Geometry check sheet. Reference: the model listing, model coordinates, mm. A direction names the side the tool comes from. Give positions to 0.01 mm unless a question says otherwise; leave off trailing zeros. Loops run counter-clockwise (first coordinate to the right, second up) from the corner with the lowest first, then second, coordinate; pieces in that order, holes last.
1. Cross-section at A-A, the plane z = 264. Record the cut outline in (x, y).
2. Release check for a two-part mould opening along X. For faces 1 (the flat face through (41, -256, 96)), 2 (the cylindrical face through (-46.583, -252.056, 269.205)), 3 (the flat face through (-26, -249, 2)) record: +X half, -X half, draft (parallel to the pull), parting line (faces both ways), or undercut.
3. Tool access check on faces 4 (the cylindrical face through (166.388, -253.042, 14.181)), 5 (the flat face through (71, -247, -22)). Record the directions out of +Z, -Z, +X, -X, +Y, -Y that give a thin tool (end or side, any length) a straight path to the whole face; none if there is none.
4. Material ranges on L1, parallel to Z at x = 88, y = -244; L2, parallel to X at y = -252.5, z = 146; L3, parallel to X at y = -245.75, z = 263.5, recorded low to high.
5. Cross-section at B-B, the plane y = -241. State how many separate pieces and enclosed holes the cut face has, plus the area to 3 significant figures.
6. Cross-section at C-C, the plane x = 38. Record the cut outline in (y, z).
7. Go/stop test with flat-tipped pins: pin 1 Ø3 at (y, z) = (-239.5, 123) entering from +X; pin 2 Ø1 at (y, z) = (-254, 139) entering from +X; pin 3 Ø6.5 at (x, z) = (-71.3, 124.3) entering from -Y. Record where each tip stops, or that it passes through.
8. Cross-section at D-D, the plane x = 138.5. Record the cut outline in (y, z), plus the area to 3 significant figures.
from build123d import *

# Parameters (mm, degrees)
SKETCH_R            = 2.75
SKETCH_R_2          = 3.2
PAD_DEPTH           = 19.05
HOLE_D              = 6.4
HOLE_CBORE_D        = 10.5
HOLE_CBORE_DEPTH    = 8
HOLE001_D           = 5.5
HOLE001_CBORE_D     = 9.5
HOLE001_CBORE_DEPTH = 6
SKETCH005_R         = 19.05
SKETCH005_R_2       = 2.1
POCKET_DEPTH        = 19.051
HOLE005_D           = 6.4
HOLE005_CBORE_D     = 10.5
HOLE005_CBORE_DEPTH = 8
SKETCH022_R         = 2.1
POCKET010_DEPTH     = 19.051
SKETCH027_R         = 2.5
POCKET013_DEPTH     = 20
SKETCH028_R         = 1.25
SKETCH028_R_2       = 3.2
POCKET014_DEPTH     = 19.051


with BuildPart() as part:
    # Sketch → Pad (new body)
    with BuildSketch(Plane.XZ):
        Polygon((-84, 276.7), (-84, 111.6), (-26, 26), (-26, -22), (170, -22), (170, 26), (-0.6, 276.7), align=None)
        with Locations((-18, 16)):
            Circle(SKETCH_R, mode=Mode.SUBTRACT)
        with Locations((18, 16)):
            Circle(SKETCH_R, mode=Mode.SUBTRACT)
        with Locations((-18, -16)):
            Circle(SKETCH_R, mode=Mode.SUBTRACT)
        with Locations((18, -16)):
            Circle(SKETCH_R, mode=Mode.SUBTRACT)
        with Locations((126, 16)):
            Circle(SKETCH_R, mode=Mode.SUBTRACT)
        with Locations((162, 16)):
            Circle(SKETCH_R, mode=Mode.SUBTRACT)
        with Locations((126, -16)):
            Circle(SKETCH_R, mode=Mode.SUBTRACT)
        with Locations((162, -16)):
            Circle(SKETCH_R, mode=Mode.SUBTRACT)
        with Locations((-71.3, 124.3)):
            Circle(SKETCH_R_2, mode=Mode.SUBTRACT)
        with Locations((-45.9, 124.3)):
            Circle(SKETCH_R_2, mode=Mode.SUBTRACT)
        with Locations((-71.3, 149.7)):
            Circle(SKETCH_R_2, mode=Mode.SUBTRACT)
        with Locations((-45.9, 149.7)):
            Circle(SKETCH_R_2, mode=Mode.SUBTRACT)
        with Locations((-71.3, 238.6)):
            Circle(SKETCH_R_2, mode=Mode.SUBTRACT)
        with Locations((-45.9, 238.6)):
            Circle(SKETCH_R_2, mode=Mode.SUBTRACT)
        with Locations((-71.3, 264)):
            Circle(SKETCH_R_2, mode=Mode.SUBTRACT)
        with Locations((-45.9, 264)):
            Circle(SKETCH_R_2, mode=Mode.SUBTRACT)
    extrude(amount=-PAD_DEPTH)

    # Hole (through all)
    with Locations(Plane.XZ):
        with Locations((-71.3, 264), (-45.9, 264), (-45.9, 238.6), (-71.3, 238.6), (-71.3, 149.7), (-45.9, 149.7), (-45.9, 124.3), (-71.3, 124.3)):
            CounterBoreHole(HOLE_D / 2, HOLE_CBORE_D / 2, HOLE_CBORE_DEPTH)

    # Hole001 (through all)
    with Locations(Plane.XZ):
        with Locations((-18, 16), (18, 16), (-18, -16), (18, -16), (126, 16), (162, 16), (126, -16), (162, -16)):
            CounterBoreHole(HOLE001_D / 2, HOLE001_CBORE_D / 2, HOLE001_CBORE_DEPTH)

    # Sketch005 (on Face4 of Hole001) → Pocket (cut, through all)
    with BuildSketch(Plane.XZ):
        with Locations((-39.95, 194.15)):
            Circle(SKETCH005_R)
        with Locations((-63.5, 217.7)):
            Circle(SKETCH005_R_2)
        with Locations((-16.4, 217.7)):
            Circle(SKETCH005_R_2)
        with Locations((-63.5, 170.6)):
            Circle(SKETCH005_R_2)
        with Locations((-16.4, 170.6)):
            Circle(SKETCH005_R_2)
    extrude(amount=-POCKET_DEPTH, mode=Mode.SUBTRACT)

    # Hole005 (through all)
    with Locations(Plane.XZ):
        with Locations((-71.3, 194.15)):
            CounterBoreHole(HOLE005_D / 2, HOLE005_CBORE_D / 2, HOLE005_CBORE_DEPTH)

    # Sketch022 (on Face4 of Hole005) → Pocket010 (cut, through all)
    with BuildSketch(Plane.XZ):
        with Locations((56, 16)):
            Circle(SKETCH022_R)
        with Locations((56, -16)):
            Circle(SKETCH022_R)
        with Locations((88, 16)):
            Circle(SKETCH022_R)
        with Locations((88, -16)):
            Circle(SKETCH022_R)
    extrude(amount=-POCKET010_DEPTH, mode=Mode.SUBTRACT)

    # Sketch027 (on Face7 of Pocket010) → Pocket013 (cut)
    with BuildSketch(Plane(origin=(-26, 0, 0), x_dir=(0, 0, -1), z_dir=(-1, 0, 0))):
        with Locations((0, -9.525)):
            Circle(SKETCH027_R)
    extrude(amount=-POCKET013_DEPTH, mode=Mode.SUBTRACT)

    # Sketch028 (on Face5 of Pocket013) → Pocket014 (cut, through all)
    with BuildSketch(Plane(origin=(0, 19.05, 0), x_dir=(1, 0, 0), z_dir=(0, 1, 0))):
        with Locations((-13, -234.7)):
            Circle(SKETCH028_R)
        with Locations((-13, -222.7)):
            Circle(SKETCH028_R)
        with Locations((-27, -228.7)):
            Circle(SKETCH028_R_2)
    extrude(amount=-POCKET014_DEPTH, mode=Mode.SUBTRACT)


with BuildPart() as part_1:
    # Body placement: moved
    add(part.part.moved(Location((0, -256, 0))))


solid = part_1.part
Result:
1. outline: (-84, -256) - (-76.55, -256) - (-76.55, -248) - (-74.5, -248) - (-74.5, -236.95) - (-84, -236.95) - close; (-68.1, -248) - (-66.05, -248) - (-66.05, -256) - (-51.15, -256) - (-51.15, -248) - (-49.1, -248) - (-49.1, -236.95) - (-68.1, -236.95) - close; (-42.7, -248) - (-40.65, -248) - (-40.65, -256) - (8.04, -256) - (8.04, -236.95) - (-42.7, -236.95) - close
2. face 1: draft
2. face 2: undercut
2. face 3: -X half
3. face 4: -Y
3. face 5: -Z, +X, -X, +Y, -Y
4. L1: z = -22 to -18.1, -13.9 to 13.9, 18.1 to 146.5
4. L2: x = -84 to -75.02, -67.58 to -49.62, -42.18 to 88.34
4. L3: x = -84 to -74.46, -68.14 to -49.06, -42.74 to 8.38
5. separate pieces: 1
5. enclosed holes: 29
5. area: 47,400 mm2
6. outline: (-256, -22) - (-236.95, -22) - (-236.95, 219.98) - (-256, 219.98) - close
7. pin 1: stops at x = 105.01
7. pin 2: stops at x = 93.44
7. pin 3: stops at y = -248
8. outline: (-256, -22) - (-236.95, -22) - (-236.95, 72.29) - (-256, 72.29) - close
8. area: 1,800 mm2
